```python
from build123d import *

# Parameters (mm, degrees)
BOSS_EXTRUDE1_DEPTH = 20
SKETCH2_W           = 5
SKETCH2_H           = 1.6
BOSS_EXTRUDE2_DEPTH = 13
SKETCH3_R           = 3.578569403
CUT_EXTRUDE1_DEPTH  = 7
BOSS_EXTRUDE3_DEPTH = 1.7
CUT_EXTRUDE2_START  = 20
SKETCH6_R           = 2.25
CUT_EXTRUDE2_DEPTH  = 22.6
CUT_EXTRUDE3_START  = 3
SKETCH7_R           = 3.8
CUT_EXTRUDE3_DEPTH  = 14.622368421
SKETCH8_R           = 1.65
CUT_EXTRUDE4_DEPTH  = 40
CUT_EXTRUDE5_DEPTH  = 17
SKETCH10_R          = 1.65
BOSS_EXTRUDE4_DEPTH = 0.2


with BuildPart() as part:
    # Sketch1 → Boss-Extrude1 (new body)
    with BuildSketch(Plane.XY):
        with BuildLine():
            Line((-9.975, 0), (9.975, 0))
            Line((9.975, 0), (9.975, 10))
            ThreePointArc((9.975, 10), (8.197090719, 14.521275434), (3.815771997, 16.620546549))
            ThreePointArc((3.815771997, 16.620546549), (3.204205313, 16.340903263), (3.110466203, 15.675))
            ThreePointArc((3.110466203, 15.675), (0, 11.175), (-3.110466203, 15.675))
            ThreePointArc((-3.110466203, 15.675), (-3.204205313, 16.340903263), (-3.815771997, 16.620546549))
            ThreePointArc((-3.815771997, 16.620546549), (-8.197090719, 14.521275434), (-9.975, 10))
            Line((-9.975, 10), (-9.975, 0))
        make_face()
    extrude(amount=BOSS_EXTRUDE1_DEPTH)

    # Sketch2 → Boss-Extrude2 (add)
    with BuildSketch(Plane.XY.offset(20)):
        with Locations((0, -0.8)):
            Rectangle(SKETCH2_W, SKETCH2_H)
    extrude(amount=-BOSS_EXTRUDE2_DEPTH)

    # Sketch3 → Cut-Extrude1 (cut)
    with BuildSketch(Plane(origin=(0, 0, 0), x_dir=(-1, 0, 0), z_dir=(0, 0, -1))):
        with Locations((0, 14.5)):
            Circle(SKETCH3_R)
    extrude(amount=-CUT_EXTRUDE1_DEPTH, mode=Mode.SUBTRACT)

    # Sketch4 → Boss-Extrude3 (add)
    with BuildSketch(Plane(origin=(0, 0, 0), x_dir=(-1, 0, 0), z_dir=(0, 0, -1))):
        with BuildLine():
            Line((-9.975, 0), (-9.975, 10))
            Line((-9.975, 10), (-9.752890248, 11.702738246))
            Line((-9.752890248, 11.702738246), (-1.415257539, 9.392452047))
            ThreePointArc((-1.415257539, 9.392452047), (0, 9.2), (1.415257539, 9.392452047))
            Line((1.415257539, 9.392452047), (9.752890248, 11.702738246))
            Line((9.752890248, 11.702738246), (9.975, 10))
            Line((9.975, 10), (9.975, 0))
            Line((9.975, 0), (-9.975, 0))
        make_face()
    extrude(amount=BOSS_EXTRUDE3_DEPTH)

    # Sketch6 → Cut-Extrude2 (cut, through all)
    with BuildSketch(Plane(origin=(0, 0, 0), x_dir=(1, 0, 0), z_dir=(0, 1, 0)).offset(CUT_EXTRUDE2_START)):
        with Locations((0, -13)):
            Circle(SKETCH6_R)
    extrude(amount=-CUT_EXTRUDE2_DEPTH, mode=Mode.SUBTRACT)

    # Sketch7 → Cut-Extrude3 (cut, through all)
    with BuildSketch(Plane(origin=(0, 0, 0), x_dir=(1, 0, 0), z_dir=(0, 1, 0)).offset(CUT_EXTRUDE3_START)):
        with Locations((0, -13)):
            Circle(SKETCH7_R)
    extrude(amount=CUT_EXTRUDE3_DEPTH, mode=Mode.SUBTRACT)

    # Sketch8 → Cut-Extrude4 (cut)
    with BuildSketch(Plane(origin=(0, 0, -1.7), x_dir=(-1, 0, 0), z_dir=(0, 0, -1))):
        with Locations((6.975, 5)):
            Circle(SKETCH8_R)
    cut_extrude4 = extrude(amount=-CUT_EXTRUDE4_DEPTH, mode=Mode.SUBTRACT)

    # Mirror1: Cut-Extrude4 across plane
    add(cut_extrude4.mirror(Plane(origin=(0, 0, 0), x_dir=(0, 0, 1), z_dir=(1, 0, 0))), mode=Mode.SUBTRACT)

    # Sketch9 → Cut-Extrude5 (cut)
    with BuildSketch(Plane.XY.offset(20)):
        with BuildLine():
            Line((-6.975, 8), (-9.975, 8))
            Line((-9.975, 8), (-9.975, 2))
            Line((-9.975, 2), (-6.975, 2))
            ThreePointArc((-6.975, 2), (-3.975, 5), (-6.975, 8))
        make_face()
    cut_extrude5 = extrude(amount=-CUT_EXTRUDE5_DEPTH, mode=Mode.SUBTRACT)

    # Sketch10 → Boss-Extrude4 (add)
    with BuildSketch(Plane.XY.offset(3)):
        with Locations((-6.975, 5)):
            Circle(SKETCH10_R)
    boss_extrude4 = extrude(amount=-BOSS_EXTRUDE4_DEPTH)

    # Mirror2: Cut-Extrude5, Boss-Extrude4 across plane
    add(cut_extrude5.mirror(Plane(origin=(0, 0, 0), x_dir=(0, 0, 1), z_dir=(1, 0, 0))), mode=Mode.SUBTRACT)
    add(boss_extrude4.mirror(Plane(origin=(0, 0, 0), x_dir=(0, 0, 1), z_dir=(1, 0, 0))))


solid = part.part
```
Build history of the part. All positions in model axes, mm. A direction names the side the tool comes from. Round coordinates to 2 decimals unless told otherwise and drop trailing zeros. Loops run counter-clockwise (first coordinate to the right, second up) from the corner with the lowest first, then second, coordinate; pieces in that order, holes last.
Item 1: Saw through at D-D (y = 5). List the corners of the cut face in (x, z) (3 decimals).
Item 2: Saw through at B-B (y = 14.5). List the corners of the cut face in (x, z) (3 decimals), then the cut area to 3 significant figures.
Item 3: Which spindle directions (+Z, -Z, +X, -X, +Y, -Y) get a long thin tool onto all of the face, cutting with end or side? Do faces 4 (the face through (3.32, 16.46, 9.86)), 5 (the face through (-6.62, 3.39, 0.52)), 6 (the face through (-7, 5, 3)), 7 (the face through (2.5, -1, 14)). Say none if no direction does.
Item 4: Saw through at A-A (x = 0). List the corners of the cut face in (y, z) (3 decimals), then the cut area to 3 significant figures.
Item 5: Two-plate mould, pull along Y, no slides. Class faces 1 (the face through (-7, 5, 2.8)), 2 (the face through (2, 3, 15)), 3 (the face through (-9.975, 8.4, 6.9)): released by +Y, released by -Y, zero draft, split by the parting line, or undercut.
Item 6: Pin check, flat tips, straight feed: P1, Ø6, axis at x = 1.5, z = 13, coming from the +Y side; P2, Ø8.5, axis at x = 0, y = 14.5, coming from the -Z side; P3, Ø2, axis at y = 14.5, z = 4, coming from the -X side; P4, Ø5, axis at x = -8, y = 5, coming from the +Z side. Stop position of each tip, or through.
Item 7: Drill centre lines: line 1 along Z through (x, y) = (0, 1.65); line 2 along Z through (x, y) = (-5, 5.25); line 3 along X through (y, z) = (13, 6.75). Where is each one in solid material? Low to high.
Worked answers:
1. outline: (-9.975, -1.7) - (-8.625, -1.7) - (-8.625, 2.8) - (-5.325, 2.8) - (-5.325, -1.7) - (5.325, -1.7) - (5.325, 2.8) - (8.625, 2.8) - (8.625, -1.7) - (9.975, -1.7) - (9.975, 3) - (3.975, 3) - (3.975, 20) - (-3.975, 20) - (-3.975, 3) - (-9.975, 3) - close; hole circle Ø7.6 at (0, 13)
2. outline: (-8.217, 0) - (-3.579, 0) - (-3.579, 7) - (-3.325, 7) - (-3.325, 11.16) arc R3.8 cw to (-3.325, 14.84) - (-3.325, 20) - (-8.217, 20) - close; (3.325, 7) - (3.579, 7) - (3.579, 0) - (8.217, 0) - (8.217, 20) - (3.325, 20) - (3.325, 14.84) arc R3.8 cw to (3.325, 11.16) - close
2. area: 190 mm2
3. face 4: +Z, -Z
3. face 5: -Z
3. face 6: +Z, -X
3. face 7: +Z, -Z, +X, -Y
4. outline: (-1.6, 7) - (0, 7) - (0, -1.7) - (9.2, -1.7) - (9.2, 0) - (10.921, 0) - (10.921, 7) - (11.175, 7) - (11.175, 9.2) - (3, 9.2) - (3, 10.75) - (-1.6, 10.75) - close; (-1.6, 15.25) - (3, 15.25) - (3, 16.8) - (11.175, 16.8) - (11.175, 20) - (-1.6, 20) - close
4. area: 175 mm2
5. face 1: undercut
5. face 2: released by +Y
5. face 3: zero draft
6. P1: stops at y = 16.62
6. P2: stops at z = 0
6. P3: stops at x = -8.98
6. P4: stops at z = 3
7. line 1: z = -1.7 to 10.75, 15.25 to 20
7. line 2: z = -1.7 to 3
7. line 3: x = -9.26 to -3.25, 3.25 to 9.26
